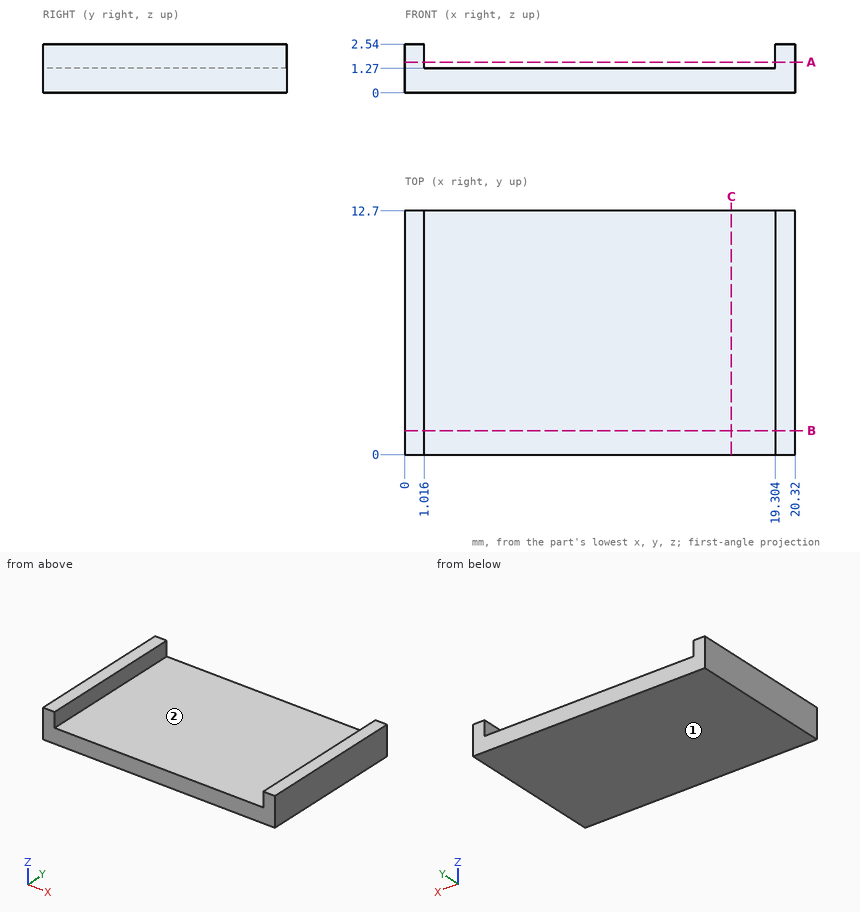
For this review, use the dimensioned drawing (mm, ordinates from the lowest corner) and the shaded views. A direction names the side the tool comes from. Round coordinates to 2 decimals unless told otherwise and drop trailing zeros. Write each loop counter-clockwise with the first axis right and the second up, starting at its lowest first coordinate (ties: lowest second). Pieces come first, ordered by that corner, then holes. Notation, with made-up numbers: M 89,64 L 109,64 A12 ccw 109,81 Z; hole C 77.25,-2.5 d3. An arc over 180 degrees is marked long. Use CSV: the item, a comma, the result in double quotes. Start each with the question number.
(1) For line 1 along X through (y, z) = (1.5, 2.45); line 2 along Z through (x, y) = (12.5, 8.25), list the stretches that pass through material, from the lowest coordinate up.
(2) We need section B-B, the plane y = 1.25. State the section outline as (x, z) points, then the cut area to 3 significant figures.
(3) We need section A-A, the plane z = 1.6. State the section outline as (x, y) points.
(4) Tool access review of the marked faces 1 and 2: name each direction out of +Z, -Z, +X, -X, +Y, -Y from which nothing blocks a thin tool from reaching the whole face with its end or side.
(5) Clearance check with a flat-ended pin moving along its axis: P1, Ø5, axis at x = 9.5, y = 7.5, coming from the +Z side. State where the tip first meets the part, or that it passes through.
(6) We need section C-C, the plane x = 17. State the section outline as (y, z) points.
Findings:
1,line 1,"0 to 1.02, 19.3 to 20.32"
1,line 2,"0 to 1.27"
2,outline,"M 0,0 L 20.32,0 L 20.32,2.54 L 19.3,2.54 L 19.3,1.27 L 1.02,1.27 L 1.02,2.54 L 0,2.54 Z"
2,area,"28.4 mm^2"
3,outline,"M 0,0 L 1.02,0 L 1.02,12.7 L 0,12.7 Z; M 19.3,0 L 20.32,0 L 20.32,12.7 L 19.3,12.7 Z"
4,face 1,"-Z, +X, -X, +Y, -Y"
4,face 2,"+Z, +Y, -Y"
5,P1,"z = 1.27"
6,outline,"M 0,0 L 12.7,0 L 12.7,1.27 L 0,1.27 Z"
